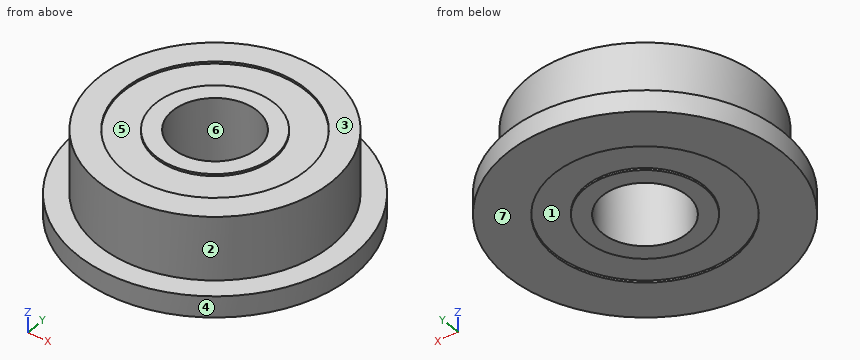
Autodesk Inventor part; units mm, degrees
ref_plane "YZ Plane" through (0, 0, 0) normal (1, 0, 0) x (0, 1, 0)
ref_plane "XZ Plane" through (0, 0, 0) normal (0, 1, 0) x (-1, 0, 0)
ref_plane "XY Plane" through (0, 0, 0) normal (0, 0, 1) x (1, 0, 0)
sketch "スケッチ1" plane through (0, 0, 0) normal (0, 0, 1) x (1, 0, 0)
  circle A0 centre (0, 0) radius 2
  circle A1 centre (0, 0) radius 5.5
  circle A2 centre (0, 0) radius 6.5
  dimension "d0" = 4
  dimension "d1" = 11
  dimension "d2" = 1
extrude "押し出し1" add sketch "スケッチ1" along normal blind 4 contours A1
extrude "押し出し2" add sketch "スケッチ1" along normal blind 1 contours A2
sketch "スケッチ2" plane through (0, 0, 0) normal (0, 0, -1) x (-1, 0, 0)
  circle A0 centre (0, 0) radius 2.8
  circle A1 centre (0, 0) radius 4.3
  dimension "d7" = 5.6
  dimension "d8" = 8.6
extrude "押し出し3" cut sketch "スケッチ2" against normal blind 0.1
sketch "スケッチ3" plane through (0, 0, 4) normal (0, 0, 1) x (1, 0, 0)
  circle A0 centre (0, 0) radius 2.8
  circle A1 centre (0, 0) radius 4.3
  dimension "d11" = 5.6
  dimension "d12" = 8.6
extrude "押し出し4" cut sketch "スケッチ3" against normal blind 0.1
properties part number "ベアリングFd4D11B4" material "鋼、炭素鋼"
Source: CAD feature listing. Evaluate the final solid. Frame: model axes, mm. Face numbers are marked on the shaded views. A direction names the side the tool comes from. Coordinates: 2 decimals unless noted, no trailing zeros. Loops run counter-clockwise (first coordinate to the right, second up) from the corner with the lowest first, then second, coordinate; pieces in that order, holes last. Notation, with made-up numbers: M 75,-25 L 93,-25 A33 ccw 93,7 Z; hole C 2,78 d4. An arc over 180 degrees is marked long. Answer in a Markdown table with one row per item.
Q1. Section C-C on z = 0.4. Return the cut outline in (x, y).
Answers below:
| item | result |
|---|---|
| outline | C 0,0 d13; hole C 0,0 d4 |
Q2. Draft query along X for the marked faces 4, 5, 6 and 7. Return one class per face: pulls with the +X half, pulls with the -X half, needs draft (parallel to the pull), parting line crosses it, or undercut.
Answers below:
| item | result |
|---|---|
| face 4 | parting line crosses it |
| face 5 | undercut |
| face 6 | undercut |
| face 7 | needs draft |
Q3. Set-up query: the marked faces 1, 2 and 3. Return all of +Z, -Z, +X, -X, +Y, -Y with unobstructed straight access to the full face (end or side cutting, diameter ignored); none if empty.
Answers below:
| item | result |
|---|---|
| face 1 | -Z |
| face 2 | +Z |
| face 3 | +Z, +X, -X, +Y, -Y |
Q4. Ray query, probe 1 along Y at (x, z) = (0, 2.3); probe 2 along Z at (x, y) = (4, -1); probe 3 along Z at (x, y) = (1, 5.5). Return the intervals inside material, ascending. Write a range as from..to.
Answers below:
| item | result |
|---|---|
| probe 1 | y = -5.5..-2, 2..5.5 |
| probe 2 | z = 0.1..3.9 |
| probe 3 | z = 0..1 |
Q5. Section D-D on y = -4.5. Return the cut outline in (x, z), plus the area to 3 significant figures.
Answers below:
| item | result |
|---|---|
| outline | M -4.69,0 L 4.69,0 L 4.69,1 L 3.16,1 L 3.16,4 L -3.16,4 L -3.16,1 L -4.69,1 Z |
| area | 28.4 mm^2 |
Q6. Section A-A on x = 0. Return the cut outline in (y, z).
Answers below:
| item | result |
|---|---|
| outline | M -6.5,0 L -4.3,0 L -4.3,0.1 L -2.8,0.1 L -2.8,0 L -2,0 L -2,4 L -2.8,4 L -2.8,3.9 L -4.3,3.9 L -4.3,4 L -5.5,4 L -5.5,1 L -6.5,1 Z; M 2,0 L 2.8,0 L 2.8,0.1 L 4.3,0.1 L 4.3,0 L 6.5,0 L 6.5,1 L 5.5,1 L 5.5,4 L 4.3,4 L 4.3,3.9 L 2.8,3.9 L 2.8,4 L 2,4 Z |
